Read the model definition and answer for the solid it produces. Units are mm, in the model's axes. A direction names the side the tool comes from. Give positions to 0.01 mm unless a question says otherwise; leave off trailing zeros. Loops run counter-clockwise (first coordinate to the right, second up) from the corner with the lowest first, then second, coordinate; pieces in that order, holes last. Notation, with made-up numbers: (69.25, 48.5) - (98.25, 48.5) arc R24 ccw to (98.25, 72.5) - close; hole circle Ø6 at (-37, -3.5). An arc over 180 degrees is marked (long way). Write item = value, one per line. Start each with the question number.
from build123d import *

# Parameters (mm, degrees)
F0_R     = 32.5
F1_DEPTH = 200
F2_R     = 15
F3_DEPTH = 50
F4_DEPTH = 250


with BuildPart() as f1:
    # F0 (on Top) → F1 (new body)
    with BuildSketch(Plane.XY):
        Circle(F0_R)
    extrude(amount=F1_DEPTH)

    # F2 (on face) → F3 (join)
    with BuildSketch(Plane.XY.offset(200)):
        Circle(F2_R)
    extrude(amount=F3_DEPTH)

    # F2 (on face) → F4 (join)
    with BuildSketch(Plane.XY.offset(200)):
        Circle(F2_R)
    extrude(amount=-F4_DEPTH)


solid = f1.part
1. Consider line 1 along Z through (x, y) = (-9, 26.5); line 2 along X through (y, z) = (2, 80); line 3 along X through (y, z) = (-0.5, 199). Determine where each line is inside the solid, lowest interval first. Write a range as [from, to].
2. A cutting plane is placed at D-D on y = -26. Give the vertices of the cut face in (x, z), and give its area (3 significant figures).
3. Given P1, Ø5, axis at x = 8.5, z = 52, coming from the -Y side; P2, Ø1.5, axis at y = 18.5, z = 75.5, coming from the +X side; P3, Ø3, axis at y = -19, z = 54, coming from the +X side, each flat-ended and moving along its own axis, determine where each tip first touches the part or whether it passes through.
4. A cutting plane is placed at C-C on z = 109. Give the vertices of the cut face in (x, y), and give its area (3 significant figures).
5. A tool of negligible diameter and unlimited length cuts with its end or side. For faces 1 (the flat face through (0, 0, 250)), 2 (the cylindrical face through (-14.985, 0.66, 224.65)), 3 (the flat face through (14, -7, 0)), from which of +Z, -Z, +X, -X, +Y, -Y can it reach the whole face along a straight path? Write none if from no direction.
6. A cutting plane is placed at A-A on y = 0. Give the vertices of the cut face in (x, z), and give its area (3 significant figures).
Reply:
q1.line_1 = [0, 200]
q1.line_2 = [-32.44, 32.44]
q1.line_3 = [-32.5, 32.5]
q2.outline = (-19.5, 0) - (19.5, 0) - (19.5, 200) - (-19.5, 200) - close
q2.area = 7,800 mm^2
q3.P1 = -31.94
q3.P2 = 27.22
q3.P3 = 27.39
q4.outline = circle Ø65 at (0, 0)
q4.area = 3,320 mm^2
q5.face_1 = +Z, +X, -X, +Y, -Y
q5.face_2 = +Z
q5.face_3 = -Z
q6.outline = (-32.5, 0) - (-15, 0) - (-15, -50) - (15, -50) - (15, 0) - (32.5, 0) - (32.5, 200) - (15, 200) - (15, 250) - (-15, 250) - (-15, 200) - (-32.5, 200) - close
q6.area = 16,000 mm^2
